```python
from build123d import *

# Parameters (mm, degrees)
SKETCH_1_W                 = 20
SKETCH_1_H                 = 10
BASEPLATE_DEPTH            = 1
EDGEFLANGE_STRIP_W         = 8
EDGEFLANGE_STRIP_H         = 1
EDGEFLANGE_STRIP_CUT_DEPTH = 20
EDGEFLANGE_DEPTH           = 20
EDGEFLANGE_FLAT_DEPTH      = 1


# Sheet-metal steps are written as plain solids
with BuildPart() as part:
    # Sketch 1 → BasePlate (new body)
    with BuildSketch(Plane.XY):
        with Locations((10, 5)):
            Rectangle(SKETCH_1_W, SKETCH_1_H)
    extrude(amount=-BASEPLATE_DEPTH)

    # EdgeFlange strip (across the edge) → EdgeFlange strip cut (cut)
    with BuildSketch(Plane(origin=(20, 10, 0), x_dir=(0, -1, 0), z_dir=(-1, 0, 0))):
        with Locations((-1, -0.5)):
            Rectangle(EDGEFLANGE_STRIP_W, EDGEFLANGE_STRIP_H)
    extrude(amount=EDGEFLANGE_STRIP_CUT_DEPTH, mode=Mode.SUBTRACT)

    # EdgeFlange bend section (across the edge) → EdgeFlange (add)
    with BuildSketch(Plane(origin=(20, 10, 0), x_dir=(0, -1, 0), z_dir=(-1, 0, 0))):
        with BuildLine():
            Line((0, 2), (1, 2))
            ThreePointArc((1, 2), (1.585786438, 0.585786438), (3, 0))
            Line((3, 0), (3, -1))
            ThreePointArc((3, -1), (0.878679656, -0.121320344), (0, 2))
        make_face()
    extrude(amount=EDGEFLANGE_DEPTH)

    # EdgeFlange profile (on flange) → EdgeFlange flat (add)
    with BuildSketch(Plane(origin=(0, 10, 0), x_dir=(-1, 0, 0), z_dir=(0, 1, 0))):
        Polygon((-20, 20), (-20, 2), (0, 2), (0, 20), (-2, 20), (-18, 20), align=None)
    extrude(amount=-EDGEFLANGE_FLAT_DEPTH)


solid = part.part
```
Could you check a few things on this model? Use its own coordinates, in mm. A direction names the side the tool comes from. Coordinates: 2 decimals unless noted, no trailing zeros. Loops run counter-clockwise (first coordinate to the right, second up) from the corner with the lowest first, then second, coordinate; pieces in that order, holes last.
1) Which directions (+Z, -Z, +X, -X, +Y, -Y) give clear straight access to the entire face, cutting with the end or side of a thin tool? Please do faces 4 (the face through (10, 9, 11)), 5 (the face through (10, 10, 11)).
Reported:
face 4: +Z, +X, -X, -Y
face 5: +Z, -Z, +X, -X, +Y
2) Thinking about a two-plate mould opening in X: for faces 1 (the face through (0, 9.5, 7.1)), 2 (the face through (9.9, 9.5, 20)), 3 (the face through (20, 9.5, 8)), which applies, released by +X, released by -X, zero draft, split by the parting line, or undercut?
Reported:
face 1: released by -X
face 2: zero draft
face 3: released by +X
3) Will these pins go through, and if not, where does the flat tip stop? pin 1 Ø6 at (y, z) = (4.5, 15) entering from +X; pin 2 Ø12 at (x, z) = (17.5, 3.5) entering from -Y; pin 3 Ø5.5 at (x, y) = (12, 3) entering from +Z.
Reported:
pin 1: passes through
pin 2: stops at y = 0
pin 3: stops at z = 0
4) Imagine slicing it at C-C (y = 6.75). List the corners of the cut face in (x, z) for me.
Reported:
outline: (0, -1) - (20, -1) - (20, 0) - (0, 0) - close
5) Imagine slicing it at B-B (z = 5.25). List the corners of the cut face in (x, y) for me, and give its area (3 significant figures).
Reported:
outline: (0, 9) - (20, 9) - (20, 10) - (0, 10) - close
area: 20.0 mm2
6) Imagine slicing it at A-A (x = 13.25). List the corners of the cut face in (y, z) for me, and give its area (3 significant figures).
Reported:
outline: (0, -1) - (7, -1) arc R3 ccw to (10, 2) - (10, 20) - (9, 20) - (9, 2) arc R2 cw to (7, 0) - (0, 0) - close
area: 28.9 mm2
7) Please list where these lines run through material, in increasing order: line 1 along Y through (x, z) = (6.75, 18.5); line 2 along Z through (x, y) = (4.75, 4.5); line 3 along Z through (x, y) = (5.25, 7.5).
Reported:
line 1: y = 9 to 10
line 2: z = -1 to 0
line 3: z = -0.96 to 0.06
